Autodesk Inventor part; units mm, degrees
ref_plane "YZ Plane" through (0, 0, 0) normal (1, 0, 0) x (0, 1, 0)
ref_plane "XZ Plane" through (0, 0, 0) normal (0, 1, 0) x (-1, 0, 0)
ref_plane "XY Plane" through (0, 0, 0) normal (0, 0, 1) x (1, 0, 0)
sketch "Sketch1" plane through (0, 0, 0) normal (0, 1, 0) x (-1, 0, 0)
  line L0 (-8.0312, -19.6194) -> (-8.0312, -0.5694)
  line L1 (-8.0312, -0.5694) -> (-34.5277, -0.5694)
  line L2 (-34.5277, -0.5694) -> (-34.5277, -28.5056)
  line L3 (18.6455, 5.0782) -> (18.6456, 5.0782)
  line L4 (-1.974, -37.6808) -> (-8.0312, -19.6194)
  line L5 (-34.5277, -28.5056) -> (-27.4611, -49.5771)
  line L6 (-1.974, -37.6808) -> (-0.9645, -40.691)
  line L7 (-27.4611, -49.5771) -> (-0.9645, -40.691)
  circle A0 centre (-21.2795, -10.9517) radius 8.7948
  line L8 (-8.0312, -0.5694) -> (-8.0312, -19.6194)
  line L9 (-8.0312, -19.6194) -> (-0.9645, -40.691)
  line L10 (-0.9645, -40.691) -> (-27.4611, -49.5771)
  line L11 (-27.4611, -49.5771) -> (-34.5277, -28.5056)
  line L12 (-34.5277, -28.5056) -> (-34.5277, -0.5694)
  line L13 (-34.5277, -0.5694) -> (-8.0312, -0.5694)
  point P0 (0, 0)
  point P1 (-21.2795, -2.1569)
  dimension "d4" = 17.5895
  dimension "d0" = 19.05
  dimension "d1" = 22.225
  dimension "d2" = 27.9469
  dimension "d3" = 26.4965
  dimension "d17" = 13.2483
  dimension "d18" = 1.5875
  dimension "d19" = 13.2483
  dimension "d20" = 10.3823
extrude "Extrusion1" add sketch "Sketch1" along normal blind 5.588
sketch "Sketch2" plane through (0, 5.588, 0) normal (0, 1, 0) x (1, 0, 0)
  line L0 (31.5176, 27.4961) -> (8.0312, 19.6194)
  line L1 (8.0312, 19.6194) -> (7.0136, 22.6537)
  line L2 (7.0136, 22.6537) -> (27.4657, 29.5128)
  line L3 (31.5176, 27.4961) -> (29.9884, 26.9832)
  line L4 (27.4657, 29.5128) -> (21.4165, 47.5499)
  line L5 (21.4165, 47.5499) -> (24.4508, 48.5676)
  line L6 (24.4508, 48.5676) -> (31.5176, 27.4961)
  line L7 (27.4611, 49.5771) -> (0.9645, 40.691)
  point P0 (0, 0)
  point P1 (0, 0)
  dimension "d10" = 3.175
  dimension "d11" = 3.2004
  dimension "d12" = 3.2004
  dimension "d15" = 0
extrude "Extrusion2" cut sketch "Sketch2" against normal blind 1.5875
fillet "Fillet1" radius 1.5875 1 edges at (31.5176, 4.7942, -27.4961)
properties part number "Lidar Sensor Case Piece 2"
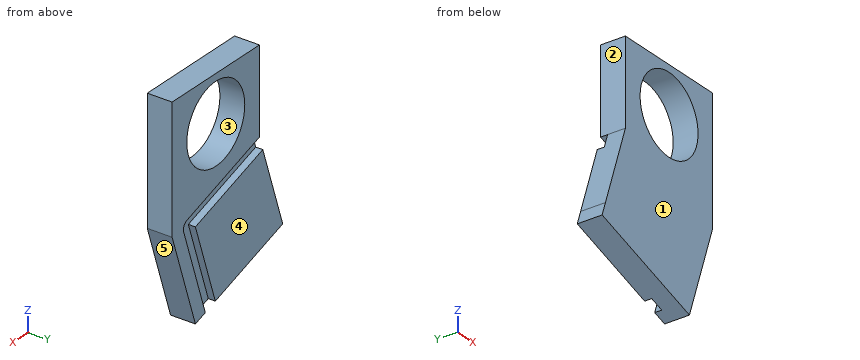
Source: CAD feature listing. Evaluate the final solid. Frame: model axes, mm. Face numbers are marked on the shaded views. A direction names the side the tool comes from. Coordinates: 2 decimals unless noted, no trailing zeros. Order: outer loops, then holes, each group sorted by start corner. A loop starts at its lowest first (then second) coordinate and runs counter-clockwise, first axis right, second up. Notation, with made-up numbers: M 89,-1 L 145,-1 A23 cw 145,34 Z; hole C 6,-5 d3. An arc over 180 degrees is marked long. Write each question's results on one line, items separated by ' | '. Start each with the question number.
1. Section B-B, the plane z = -5. Return the cut outline in (x, y).
2. Pin query (flat end, axial travel): pin 1 (14 mm diameter, centred on x = 21.28, z = -10.95, fed in from +Y). Return the tip coordinate at first contact, or that it passes through.
3. Reachability of the marked faces 1 and 2 from +Z, -Z, +X, -X, +Y, -Y: full face, straight path, thin tool, end or side. Return the list, or none.
4. Section A-A, the plane y = 4.6. Return the cut outline in (x, z) (1 decimal), then the cut area to 3 significant figures.
5. Section C-C, the plane z = -27.5. Return the cut outline in (x, y), then the cut area to 3 significant figures.
6. Draft query along X for the marked faces 3, 4 and 5. Return one class per face: +X half, -X half, draft (parallel to the pull), parting line (faces both ways), or undercut.
7. Material intervals for L1, parallel to Z at x = 20, y = 4.95; L2, parallel to X at y = 2.35, z = -11; L3, parallel to X at y = 1.5, z = -17.5, sorted ascending.
8. Section D-D, the plane x = 11.5. Return the cut outline in (y, z), then the cut area to 3 significant figures.
Solution:
1) outline: M 8.03,0 L 14.8,0 L 14.8,5.59 L 8.03,5.59 Z; M 27.75,0 L 34.53,0 L 34.53,5.59 L 27.75,5.59 Z
2) pin 1: through
3) face 1: +Z, -Z, +X, -X, -Y | face 2: +Z, -X, +Y, -Y
4) outline: M 1,-40.7 L 21.4,-47.5 L 27.5,-29.5 L 7,-22.7 L 2,-37.7 Z; M 8,-19.6 L 30,-27 A1.6 cw 31,-29 L 24.5,-48.6 L 27.5,-49.6 L 34.5,-28.5 L 34.5,-0.6 L 8,-0.6 Z; hole C 21.3,-11 d17.6 | area: 861 mm²
5) outline: M 5.39,0 L 34.53,0 L 34.53,5.59 L 30.74,5.59 L 30.74,4 L 21.46,4 L 21.46,5.59 L 5.39,5.59 Z | area: 148 mm²
6) face 3: undercut | face 4: draft | face 5: +X half
7) L1: -47.07 to -27.01, -23.63 to -19.65, -2.25 to -0.57 | L2: 8.03 to 12.48, 30.07 to 34.53 | L3: 8.03 to 15.41, 27.15 to 34.53
8) outline: M 0,-44.22 L 5.59,-44.22 L 5.59,-24.16 L 4,-24.16 L 4,-20.78 L 5.59,-20.78 L 5.59,-0.57 L 0,-0.57 Z | area: 239 mm²
